```python
from build123d import *

# Parameters (mm, degrees)
SKETCH_1_W               = 60
SKETCH_1_H               = 45
EXTRUDE_1_DEPTH          = 60
SKETCH_3_R               = 4
CUT_EXTRUDE_1_DEPTH      = 1
CUT_EXTRUDE_1_DEPTH_BACK = 46
SKETCH_4_R               = 3
CUT_EXTRUDE_2_DEPTH      = 1
CUT_EXTRUDE_2_DEPTH_BACK = 61
CUT_EXTRUDE_8_DEPTH      = 7.2
CUT_EXTRUDE_9_REACH      = 54.194
SKETCH_6_W               = 14.4
SKETCH_6_H               = 6.7


with BuildPart() as part:
    # 스케치1 → 보스-돌출1 (new body)
    with BuildSketch(Plane.XY):
        Rectangle(SKETCH_1_W, SKETCH_1_H)
    extrude(amount=EXTRUDE_1_DEPTH)

    # 스케치2 → 컷-회전1 (revolve, cut)
    with BuildSketch(Plane(origin=(0, 0, 30), x_dir=(-1, 0, 0), z_dir=(0, 0, -1))):
        Polygon((0, 17.5), (0, -22.5), (-27, -22.5), align=None)
    revolve(axis=Axis((0, 17.5, 30), (0, -1, 0)), mode=Mode.SUBTRACT)

    # 스케치3 → 컷-돌출1 (cut, two sides)
    with BuildSketch(Plane(origin=(0, 22.5, 0), x_dir=(1, 0, 0), z_dir=(0, 1, 0))) as cut_extrude_1_sk:
        with Locations((0, -30)):
            Circle(SKETCH_3_R)
    extrude(amount=CUT_EXTRUDE_1_DEPTH, mode=Mode.SUBTRACT)
    extrude(cut_extrude_1_sk.sketch, amount=-CUT_EXTRUDE_1_DEPTH_BACK, mode=Mode.SUBTRACT)

    # 스케치4 → 컷-돌출2 (cut, two sides)
    with BuildSketch(Plane(origin=(0, 0, 0), x_dir=(-1, 0, 0), z_dir=(0, 0, -1))) as cut_extrude_2_sk:
        with Locations((-25.9, 18.4)):
            Circle(SKETCH_4_R)
        with Locations((-25.9, 2.5)):
            Circle(SKETCH_4_R)
        with Locations((-9.1, 18.4)):
            Circle(SKETCH_4_R)
        with Locations((-9.1, 2.5)):
            Circle(SKETCH_4_R)
    extrude(amount=CUT_EXTRUDE_2_DEPTH, mode=Mode.SUBTRACT)
    extrude(cut_extrude_2_sk.sketch, amount=-CUT_EXTRUDE_2_DEPTH_BACK, mode=Mode.SUBTRACT)

    # 스케치5 → 컷-돌출8 (cut, symmetric)
    with BuildSketch(Plane(origin=(0, 0, 30), x_dir=(-1, 0, 0), z_dir=(0, 0, -1))):
        Polygon((15.370551943, 3.576426178), (27.958691181, -15.072668989), (30, -13.694785536), (30, 22.5), (11.174505531, 9.792791233), align=None)
    extrude(amount=CUT_EXTRUDE_8_DEPTH, both=True, mode=Mode.SUBTRACT)

    # 스케치6 → 컷-돌출9 (cut, up to next)
    with BuildSketch(Plane(origin=(-12.217871783, 8.247063453, 0), x_dir=(0, 0, 1), z_dir=(-0.828848674, 0.559472855, 0)), mode=Mode.PRIVATE) as cut_extrude_9_sk1:
        with Locations((30, -1.485090483)):
            Rectangle(SKETCH_6_W, SKETCH_6_H)
    cut_extrude_9_tool1 = extrude(cut_extrude_9_sk1.sketch, amount=-CUT_EXTRUDE_9_REACH, mode=Mode.PRIVATE) & part.part
    add(cut_extrude_9_tool1.solids().sort_by_distance((-13.04874, 7.016148, 30))[0], mode=Mode.SUBTRACT)


solid = part.part
```
Can you work these out from the model? Positions are in its coordinate system, mm. A direction names the side the tool comes from. Give positions to 0.01 mm unless a question says otherwise; leave off trailing zeros. Loops run counter-clockwise (first coordinate to the right, second up) from the corner with the lowest first, then second, coordinate; pieces in that order, holes last. Notation, with made-up numbers: M -2.75,13 L 51.25,13 A21 cw 51.25,35 Z; hole C 34,24.5 d3. An arc over 180 degrees is marked long. Answer in a Markdown table with one row per item.
1. For pin 1 Ø12 at (x, y) = (20.5, -10) entering from -Z; pin 2 Ø9 at (x, z) = (0, 30) entering from -Y; pin 3 Ø1 at (x, z) = (4.5, 16.5) entering from -Y, each with a flat end and sliding along its axis, tell me the tip position at first contact or that it passes through.
Taken from the geometry:
| item | result |
|---|---|
| pin 1 | stops at z = 0 |
| pin 2 | stops at y = 10.83 |
| pin 3 | stops at y = -4.32 |
2. Thinking about a two-plate mould opening in Y: for faces 3 (the flat face through (-27, -22.5, 23)), 4 (the flat face through (0, 0, 60)), 5 (the flat face through (-12.7, 2.74, 29.9)), which applies, released by +Y, released by -Y, zero draft, split by the parting line, or undercut?
Taken from the geometry:
| item | result |
|---|---|
| face 3 | released by -Y |
| face 4 | zero draft |
| face 5 | undercut |
3. If I drill on line 1 along Z through (x, y) = (0, 19); line 2 along X through (y, z) = (20, 30); line 3 along X through (y, z) = (16, 29), over which ranges is the centre line in solid material (lowest first)?
Taken from the geometry:
| item | result |
|---|---|
| line 1 | z = 0 to 26, 34 to 60 |
| line 2 | x = -26.3 to -4, 4 to 6.56, 11.64 to 23.36, 28.44 to 30 |
| line 3 | x = -20.37 to -3.87, 3.87 to 7.3, 10.9 to 24.1, 27.7 to 30 |
4. Suppose I cut it at A-A on x = 0. Write out the boundary of the cut face in (y, z), plus the area to 3 significant figures.
Taken from the geometry:
| item | result |
|---|---|
| outline | M -22.5,0 L 22.5,0 L 22.5,26 L 11.57,26 L -22.5,3 Z; M -22.5,57 L 11.57,34 L 22.5,34 L 22.5,60 L -22.5,60 Z |
| area | 1,560 mm² |
5. Suppose I cut it at D-D on y = -2.5. Write out the boundary of the cut face in (x, z), plus the area to 3 significant figures.
Taken from the geometry:
| item | result |
|---|---|
| outline | M -30,0 L 30,0 L 30,60 L -30,60 L -30,37.2 L -19.47,37.2 L -19.47,22.8 L -30,22.8 Z; hole C 0,30 d27 |
| area | 2,880 mm² |
6. Suppose I cut it at C-C on z = 30. Write out the boundary of the cut face in (x, y).
Taken from the geometry:
| item | result |
|---|---|
| outline | M -30,-22.5 L -27,-22.5 L -10.82,1.47 L -14.92,4.24 L -27.96,-15.07 L -30,-13.69 Z; M -30,22.5 L -7.07,7.02 L -4,11.57 L -4,22.5 Z; M 4,11.57 L 8.19,5.36 A3 cw 11.41,0.59 L 27,-22.5 L 30,-22.5 L 30,22.5 L 4,22.5 Z; hole C 9.1,18.4 d6; hole C 25.9,2.5 d6; hole C 25.9,18.4 d6 |
7. Suppose I cut it at B-B on y = 17. Write out the boundary of the cut face in (x, z).
Taken from the geometry:
| item | result |
|---|---|
| outline | M -30,0 L 6.45,0 L 6.45,60 L -30,60 L -30,37.2 L -21.85,37.2 L -21.85,22.8 L -30,22.8 Z; M 11.75,0 L 23.25,0 L 23.25,60 L 11.75,60 Z; M 28.55,0 L 30,0 L 30,60 L 28.55,60 Z; hole C 0,30 d8 |
8. Which directions (+Z, -Z, +X, -X, +Y, -Y) give clear straight access to the entire face, cutting with the end or side of a thin tool? Please do faces 1 (the flat face through (-28.97, -14.39, 29.9)), 2 (the flat face through (30, 0, 30)).
Taken from the geometry:
| item | result |
|---|---|
| face 1 | none |
| face 2 | +Z, -Z, +X, +Y, -Y |
